The listing builds one solid part. Answer for the finished solid, in the listing's coordinates (mm). Face numbers are marked on the shaded views. A direction names the side the tool comes from. Give positions to 0.01 mm unless a question says otherwise; leave off trailing zeros. Loops run counter-clockwise (first coordinate to the right, second up) from the corner with the lowest first, then second, coordinate; pieces in that order, holes last. Notation, with made-up numbers: M 64,87.5 L 100,87.5 A13 ccw 100,91.5 Z; hole C 2.25,44.5 d7. An arc over 180 degrees is marked long. Return JSON: item names as keys, results as strings.
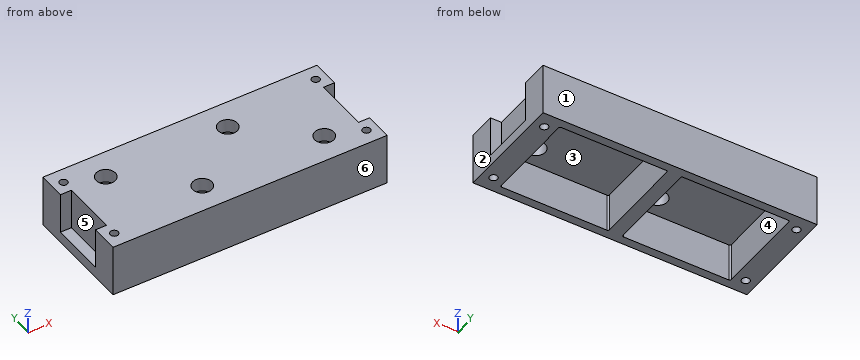
from build123d import *

# Parameters (mm, degrees)
SKETCH1_W           = 100
SKETCH1_H           = 40
BOSS_EXTRUDE1_DEPTH = 38
CUT_EXTRUDE2_START  = -12
SKETCH2_W           = 39.5
SKETCH2_H           = 34
CUT_EXTRUDE2_DEPTH  = 21
CUT_EXTRUDE3_DEPTH  = 9
CUT_EXTRUDE4_REACH  = 81.36
SKETCH4_R           = 1.45
SKETCH5_W           = 100
SKETCH5_H           = 19
CUT_EXTRUDE5_DEPTH  = 87.215210375
FILLET1_R           = 0.5
CUT_EXTRUDE11_REACH = 73.063
SKETCH10_R          = 3.5
SKETCH11_W          = 4
SKETCH11_H          = 20
CUT_EXTRUDE12_DEPTH = 15


with BuildPart() as part:
    # Sketch1 → Boss-Extrude1 (new body)
    with BuildSketch(Plane.XY):
        with Locations((16.25, 1.5625)):
            Rectangle(SKETCH1_W, SKETCH1_H)
    extrude(amount=BOSS_EXTRUDE1_DEPTH)

    # Sketch2 → Cut-Extrude2 (cut)
    with BuildSketch(Plane(origin=(0, 0, 0), x_dir=(-1, 0, 0), z_dir=(0, 0, -1)).offset(CUT_EXTRUDE2_START)):
        with Locations((-38.5, 1.5625)):
            Rectangle(SKETCH2_W, SKETCH2_H)
        with Locations((6, 1.5625)):
            Rectangle(SKETCH2_W, SKETCH2_H)
    extrude(amount=-CUT_EXTRUDE2_DEPTH, mode=Mode.SUBTRACT)

    # Sketch3 → Cut-Extrude3 (cut)
    with BuildSketch(Plane(origin=(-3.362318072, 0, 0), x_dir=(-1, 0, 0), z_dir=(0, 0, -1))):
        with BuildLine():
            ThreePointArc((-61.593370612, 1.614325749), (-20.676836723, -17.421621422), (21.715969185, -1.949710178))
            ThreePointArc((21.715969185, -1.949710178), (22.204299442, 9.465009595), (10.78957967, 9.953339852))
            ThreePointArc((10.78957967, 9.953339852), (-19.986233449, -1.278769909), (-49.690320582, 12.540715264))
            ThreePointArc((-49.690320582, 12.540715264), (-61.105040355, 13.029045522), (-61.593370612, 1.614325749))
        make_face()
    extrude(amount=-CUT_EXTRUDE3_DEPTH, mode=Mode.SUBTRACT)

    # Sketch4 → Cut-Extrude4 (cut, up to next)
    with BuildSketch(Plane(origin=(0, 0, 0), x_dir=(-1, 0, 0), z_dir=(0, 0, -1)), mode=Mode.PRIVATE) as cut_extrude4_sk1:
        with Locations((-62.25, 16.0625)):
            Circle(SKETCH4_R)
    cut_extrude4_tool1 = extrude(cut_extrude4_sk1.sketch, amount=-CUT_EXTRUDE4_REACH, mode=Mode.PRIVATE) & part.part
    # Sketch4 → Cut-Extrude4 (cut, up to next)
    with BuildSketch(Plane(origin=(0, 0, 0), x_dir=(-1, 0, 0), z_dir=(0, 0, -1)), mode=Mode.PRIVATE) as cut_extrude4_sk2:
        with Locations((-62.25, -12.9375)):
            Circle(SKETCH4_R)
    cut_extrude4_tool2 = extrude(cut_extrude4_sk2.sketch, amount=-CUT_EXTRUDE4_REACH, mode=Mode.PRIVATE) & part.part
    # Sketch4 → Cut-Extrude4 (cut, up to next)
    with BuildSketch(Plane(origin=(0, 0, 0), x_dir=(-1, 0, 0), z_dir=(0, 0, -1)), mode=Mode.PRIVATE) as cut_extrude4_sk3:
        with Locations((29.75, 16.0625)):
            Circle(SKETCH4_R)
    cut_extrude4_tool3 = extrude(cut_extrude4_sk3.sketch, amount=-CUT_EXTRUDE4_REACH, mode=Mode.PRIVATE) & part.part
    # Sketch4 → Cut-Extrude4 (cut, up to next)
    with BuildSketch(Plane(origin=(0, 0, 0), x_dir=(-1, 0, 0), z_dir=(0, 0, -1)), mode=Mode.PRIVATE) as cut_extrude4_sk4:
        with Locations((29.75, -12.9375)):
            Circle(SKETCH4_R)
    cut_extrude4_tool4 = extrude(cut_extrude4_sk4.sketch, amount=-CUT_EXTRUDE4_REACH, mode=Mode.PRIVATE) & part.part
    add(cut_extrude4_tool1.solids().sort_by_distance((62.25, 16.0625, 0))[0], mode=Mode.SUBTRACT)
    add(cut_extrude4_tool2.solids().sort_by_distance((62.25, -12.9375, 0))[0], mode=Mode.SUBTRACT)
    add(cut_extrude4_tool3.solids().sort_by_distance((-29.75, 16.0625, 0))[0], mode=Mode.SUBTRACT)
    add(cut_extrude4_tool4.solids().sort_by_distance((-29.75, -12.9375, 0))[0], mode=Mode.SUBTRACT)

    # Sketch5 → Cut-Extrude5 (cut, through all)
    with BuildSketch(Plane(origin=(0, 21.5625, 0), x_dir=(1, 0, 0), z_dir=(0, 1, 0))):
        with Locations((16.25, -9.5)):
            Rectangle(SKETCH5_W, SKETCH5_H)
    extrude(amount=-CUT_EXTRUDE5_DEPTH, mode=Mode.SUBTRACT)

    # Fillet1
    fillet1_edges = [part.edges().sort_by_distance(p)[0] for p in [
        (58.25, 18.5625, 26),
        (18.75, 18.5625, 26),
        (18.75, -15.4375, 26),
        (58.25, -15.4375, 26),
        (13.75, 18.5625, 26),
        (-25.75, 18.5625, 26),
        (-25.75, -15.4375, 26),
        (13.75, -15.4375, 26),
    ]]
    fillet(fillet1_edges, radius=FILLET1_R)

    # Sketch10 → Cut-Extrude11 (cut, up to next)
    with BuildSketch(Plane(origin=(0, 0, 33), x_dir=(-1, 0, 0), z_dir=(0, 0, -1)), mode=Mode.PRIVATE) as cut_extrude11_sk1:
        with Locations((-49.860388068, -8.232477434)):
            Circle(SKETCH10_R)
    cut_extrude11_tool1 = extrude(cut_extrude11_sk1.sketch, amount=-CUT_EXTRUDE11_REACH, mode=Mode.PRIVATE) & part.part
    # Sketch10 → Cut-Extrude11 (cut, up to next)
    with BuildSketch(Plane(origin=(0, 0, 33), x_dir=(-1, 0, 0), z_dir=(0, 0, -1)), mode=Mode.PRIVATE) as cut_extrude11_sk2:
        with Locations((-27.139611932, 11.357477434)):
            Circle(SKETCH10_R)
    cut_extrude11_tool2 = extrude(cut_extrude11_sk2.sketch, amount=-CUT_EXTRUDE11_REACH, mode=Mode.PRIVATE) & part.part
    # Sketch10 → Cut-Extrude11 (cut, up to next)
    with BuildSketch(Plane(origin=(0, 0, 33), x_dir=(-1, 0, 0), z_dir=(0, 0, -1)), mode=Mode.PRIVATE) as cut_extrude11_sk3:
        with Locations((-5.360388068, -8.232477434)):
            Circle(SKETCH10_R)
    cut_extrude11_tool3 = extrude(cut_extrude11_sk3.sketch, amount=-CUT_EXTRUDE11_REACH, mode=Mode.PRIVATE) & part.part
    # Sketch10 → Cut-Extrude11 (cut, up to next)
    with BuildSketch(Plane(origin=(0, 0, 33), x_dir=(-1, 0, 0), z_dir=(0, 0, -1)), mode=Mode.PRIVATE) as cut_extrude11_sk4:
        with Locations((17.360388068, 11.357477434)):
            Circle(SKETCH10_R)
    cut_extrude11_tool4 = extrude(cut_extrude11_sk4.sketch, amount=-CUT_EXTRUDE11_REACH, mode=Mode.PRIVATE) & part.part
    add(cut_extrude11_tool1.solids().sort_by_distance((49.860388, -8.232477, 33))[0], mode=Mode.SUBTRACT)
    add(cut_extrude11_tool2.solids().sort_by_distance((27.139612, 11.357477, 33))[0], mode=Mode.SUBTRACT)
    add(cut_extrude11_tool3.solids().sort_by_distance((5.360388, -8.232477, 33))[0], mode=Mode.SUBTRACT)
    add(cut_extrude11_tool4.solids().sort_by_distance((-17.360388, 11.357477, 33))[0], mode=Mode.SUBTRACT)

    # Sketch11 → Cut-Extrude12 (cut)
    with BuildSketch(Plane.XY.offset(38)):
        with Locations((-31.75, 1.5625)):
            Rectangle(SKETCH11_W, SKETCH11_H)
        with Locations((64.25, 1.5625)):
            Rectangle(SKETCH11_W, SKETCH11_H)
    extrude(amount=-CUT_EXTRUDE12_DEPTH, mode=Mode.SUBTRACT)


solid = part.part
(1) The part is cut by section B-B (x = 0.5). Determine the outline of the cut face in (y, z).
Values follow:
{"outline": "M -18.44,19 L -15.44,19 L -15.44,33 L 18.56,33 L 18.56,19 L 21.56,19 L 21.56,38 L -18.44,38 Z"}
(2) A tool of negligible diameter and unlimited length cuts with its end or side. For the marked faces 4, 5 and 6, from which of +Z, -Z, +X, -X, +Y, -Y can it reach the whole face along a straight path? Write none if from no direction.
Values follow:
{"face 4": "-Z", "face 5": "+Z, -X", "face 6": "+Z, -Z, +X, -X, -Y"}
(3) The part is cut by section C-C (y = 0). Determine the outline of the cut face in (x, z).
Values follow:
{"outline": "M -33.75,19 L -25.75,19 L -25.75,33 L 13.75,33 L 13.75,19 L 18.75,19 L 18.75,33 L 58.25,33 L 58.25,19 L 66.25,19 L 66.25,23 L 62.25,23 L 62.25,38 L -29.75,38 L -29.75,23 L -33.75,23 Z"}
(4) The part is cut by section D-D (z = 27.75). Give the number of separate pieces and of enclosed holes in the cut face, and give its area (3 significant figures).
Values follow:
{"separate pieces": "1", "enclosed holes": "6", "area": "1,130 mm²"}
(5) Straight lines are drawn through the part: line 1 along X through (y, z) = (-3, 32.5); line 2 along X through (y, z) = (-14.5, 21.5); line 3 along Y through (x, z) = (29, 30.25). For each, find the intervals that lie inside material, in ascending order.
Values follow:
{"line 1": "-29.75 to -25.75, 13.75 to 18.75, 58.25 to 62.25", "line 2": "-33.75 to -25.75, 13.75 to 18.75, 58.25 to 66.25", "line 3": "-18.44 to -15.44, 18.56 to 21.56"}
(6) Determine the mould class of the marked faces 1, 2 and 3 for opening direction X: released by +X, released by -X, zero draft, split by the parting line, or undercut.
Values follow:
{"face 1": "zero draft", "face 2": "released by +X", "face 3": "undercut"}
(7) Given pin 1 (1.5 mm diameter, centred on y = -0.5, z = 25.5, fed in from -X); pin 2 (4.5 mm diameter, centred on y = -2.5, z = 30, fed in from +X); pin 3 (1 mm diameter, centred on x = -18, y = -13, fed in from -Z), each flat-ended and moving along its own axis, determine where each tip first touches the part or whether it passes through.
Values follow:
{"pin 1": "x = -29.75", "pin 2": "x = 62.25", "pin 3": "z = 33"}
(8) The part is cut by section A-A (x = 50). Determine the outline of the cut face in (y, z), and give its area (3 significant figures).
Values follow:
{"outline": "M -18.44,19 L -15.44,19 L -15.44,33 L -11.73,33 L -11.73,38 L -18.44,38 Z; M -4.74,33 L 18.56,33 L 18.56,19 L 21.56,19 L 21.56,38 L -4.74,38 Z", "area": "249 mm²"}
